Autodesk Inventor part; units mm, degrees
ref_plane "Work Plane1" through (0, 0, 1.5875) normal (0, 0, -1) x (-1, 0, 0)
ref_plane "Work Plane2" through (0, 0, 100.965) normal (0, 0, 1) x (1, 0, 0)
ref_plane "Work Plane3" through (0, 0, 128.5875) normal (0, 0, 1) x (1, 0, 0)
sketch "Sketch1" plane through (0, 0, 0) normal (0, 0, 1) x (1, 0, 0)
  arc A0 (-1, 4.6563) -> (1, 4.6563) centre (0, 0) ccw
  line L0 (-1, 3.7625) -> (1, 3.7625)
  line L1 (1, 3.7625) -> (1, 4.6563)
  line L2 (1, 5.7625) -> (-1, 5.7625) construction
  line L3 (-1, 5.7625) -> (-1, 4.6563) construction
  arc A1 (1, 4.6563) -> (-1, 4.6563) centre (0, 0) ccw construction
  line L4 (-1, 4.6563) -> (-1, 3.7625)
  line L5 (1, 4.6563) -> (1, 5.7625) construction
  dimension "d0" = 9.525
  dimension "d3" = 2
  dimension "d4" = 2
  dimension "d5" = 1
  dimension "d6" = 3.7625
extrude "Extrusion1" add sketch "Sketch1" along normal blind 130.175
ref_plane "Work Plane1" through (0, 0, 1.5875) normal (0, 0, -1) x (-1, 0, 0)
sketch "Sketch2" plane through (0, 0, 1.5875) normal (0, 0, -1) x (-1, 0, 0)
  line L0 (-1, 3.7625) -> (-1, 4.6563)
  line L1 (1, 3.7625) -> (-1, 3.7625)
  line L2 (1, 4.6563) -> (1, 3.7625)
  arc A0 (-1, 4.6563) -> (1, 4.6563) centre (0, 0) ccw
  arc A1 (-1, 3.8735) -> (1, 3.8735) centre (0, 0) ccw
  arc A2 (1, 3.8735) -> (-1, 3.8735) centre (0, 0) ccw construction
  dimension "d9" = 0.762
extrude "Extrusion2" cut sketch "Sketch2" against normal blind 0.762 contours A1 L2 A0 L0
ref_plane "Work Plane2" through (0, 0, 100.965) normal (0, 0, 1) x (1, 0, 0)
sketch "Sketch3" plane through (0, 0, 100.965) normal (0, 0, 1) x (1, 0, 0)
  arc A0 (1, 3.8735) -> (-1, 3.8735) centre (0, 0) ccw
  line L0 (1, 3.7625) -> (1, 4.6563)
  arc A1 (1, 4.6563) -> (-1, 4.6563) centre (0, 0) ccw
  line L1 (-1, 4.6563) -> (-1, 3.7625)
  line L2 (-1, 3.7625) -> (1, 3.7625)
  arc A2 (-1, 3.8735) -> (1, 3.8735) centre (0, 0) ccw
  arc A3 (-1, 4.6563) -> (1, 4.6563) centre (0, 0) ccw
extrude "Extrusion3" cut sketch "Sketch3" against normal blind 0.762 contours A0 L1 A1 L0 | L0 A3 L1 A2
ref_plane "Work Plane3" through (0, 0, 128.5875) normal (0, 0, 1) x (1, 0, 0)
sketch "Sketch4" plane through (0, 0, 128.5875) normal (0, 0, 1) x (1, 0, 0)
  arc A0 (-1, 3.8735) -> (1, 3.8735) centre (0, 0) ccw
  line L0 (-1, 3.7625) -> (1, 3.7625)
  line L1 (-1, 4.6563) -> (-1, 3.7625)
  line L2 (1, 3.7625) -> (1, 4.6563)
  arc A1 (-1, 4.6563) -> (1, 4.6563) centre (0, 0) ccw
extrude "Extrusion4" cut sketch "Sketch4" against normal blind 1.016 contours A0 L2 A1 L1
equation "\"d4\" = d3"
properties part number "vertical drive shaft 4"
Design review of the part built by this model. Coordinates are the model's own, in mm. A direction names the side the tool comes from. Round coordinates to 2 decimals unless told otherwise and drop trailing zeros. Order: outer loops, then holes, each group sorted by start corner. A loop starts at its lowest first (then second) coordinate and runs counter-clockwise, first axis right, second up. Notation, with made-up numbers: (-21, 81.25) - (29, 81.25) arc R19 ccw to (29, 110.25) - close; hole circle Ø10 at (89.5, -34). An arc over 180 degrees is marked (long way). One line per question, with ' | ' between items.
Item 1: Take a section at A-A, the plane x = 2.5. Write out the cut boundary in (y, z) (1 decimal), then the cut area to 3 significant figures.
Checks:
outline: (-4.1, 0) - (4.1, 0) - (4.1, 1.6) - (3.1, 1.6) - (3.1, 2.3) - (4.1, 2.3) - (4.1, 100.2) - (3.1, 100.2) - (3.1, 101) - (4.1, 101) - (4.1, 127.6) - (3.1, 127.6) - (3.1, 128.6) - (4.1, 128.6) - (4.1, 130.2) - (-4.1, 130.2) - (-4.1, 128.6) - (-3.1, 128.6) - (-3.1, 127.6) - (-4.1, 127.6) - (-4.1, 101) - (-3.1, 101) - (-3.1, 100.2) - (-4.1, 100.2) - (-4.1, 2.3) - (-3.1, 2.3) - (-3.1, 1.6) - (-4.1, 1.6) - close | area: 1,050 mm²
Item 2: Draft analysis for pull direction X (two halves, no side actions). For faces 3 (the face through (0, 0, 130.175)), 4 (the face through (0.2, -4.76, 0.78)), 5 (the face through (0, 3.762, 64)), state which applies: +X half, -X half, draft (parallel to the pull), parting line (faces both ways), or undercut.
Checks:
face 3: draft | face 4: parting line | face 5: undercut
Item 3: Take a section at B-B, the plane y = -2. Write out the cut boundary in (x, z) (1 decimal), then the cut area to 3 significant figures.
Checks:
outline: (-4.3, 0) - (4.3, 0) - (4.3, 1.6) - (3.5, 1.6) - (3.5, 2.3) - (4.3, 2.3) - (4.3, 100.2) - (3.5, 100.2) - (3.5, 101) - (4.3, 101) - (4.3, 127.6) - (3.5, 127.6) - (3.5, 128.6) - (4.3, 128.6) - (4.3, 130.2) - (-4.3, 130.2) - (-4.3, 128.6) - (-3.5, 128.6) - (-3.5, 127.6) - (-4.3, 127.6) - (-4.3, 101) - (-3.5, 101) - (-3.5, 100.2) - (-4.3, 100.2) - (-4.3, 2.3) - (-3.5, 2.3) - (-3.5, 1.6) - (-4.3, 1.6) - close | area: 1,120 mm²
Item 4: For P1, Ø1, axis at y = 4.5, z = 80, coming from the +X side; P2, Ø0.6, axis at x = 0, z = 61.5, coming from the +Y side; P3, Ø4, axis at y = -3, z = 89, coming from the -X side, all flat-tipped, find the tip position at first contact; note any pin that passes through.
Checks:
P1: x = 2.58 | P2: y = 3.76 | P3: x = -4.66
Item 5: Wall thickness on line 1 (Z direction, x = -4.5, y = 1.25) (1 decimal); line 2 (X direction, y = -0.5, z = 27); line 3 (Y direction, x = 0.5, z = 83.5): over which ranges is each line inside the solid? List them lowest first. Write a range as [from, to].
Checks:
line 1: [0, 1.6], [2.3, 100.2], [101, 127.6], [128.6, 130.2] | line 2: [-4.74, 4.74] | line 3: [-4.74, 3.76]
Item 6: Machinability: for faces 1 (the face through (-0.162, -3.997, 100.589)), 2 (the face through (0.2, -4.76, 50.59)), which of the approach directions +Z, -Z, +X, -X, +Y, -Y give a long, thin tool a straight path to every point of the face, cutting with its end or side? Answer none if there is none.
Checks:
face 1: none | face 2: +Z, -Z
Item 7: Take a section at C-C, the plane z = 67. Write out the cut boundary in (x, y).
Checks:
outline: (-1, 3.76) - (-1, 4.66) arc R4.76 ccw (long way) to (1, 4.66) - (1, 3.76) - close
